```python
from build123d import *

# Parameters (mm, degrees)
F1_W     = 170
F1_H     = 100
F1_R     = 1.75
F2_DEPTH = 5
F3_W     = 5
F3_H     = 5
F3_R     = 1.75
F4_DEPTH = 5


with BuildPart() as f2:
    # F1 (on Top) → F2 (new body)
    with BuildSketch(Plane.XY):
        with Locations((41.5, 26.75)):
            Rectangle(F1_W, F1_H)
        with Locations((14.2, 2.6)):
            Circle(F1_R, mode=Mode.SUBTRACT)
        with Locations((66.5, 7.5)):
            Circle(F1_R, mode=Mode.SUBTRACT)
        with Locations((96.5, 2.6)):
            Circle(F1_R, mode=Mode.SUBTRACT)
        with Locations((15.6, 50.9)):
            Circle(F1_R, mode=Mode.SUBTRACT)
        with Locations((66.5, 35.7)):
            Circle(F1_R, mode=Mode.SUBTRACT)
        with Locations((90.5, 50.9)):
            Circle(F1_R, mode=Mode.SUBTRACT)
    extrude(amount=F2_DEPTH)

    # F3 (on face) → F4 (cut, through all)
    with BuildSketch(Plane.XY.offset(5)):
        with Locations((-26, -20.75)):
            Rectangle(F3_W, F3_H)
        with Locations((-1, -20.75)):
            Rectangle(F3_W, F3_H)
        with Locations((-13.5, -20.75)):
            Circle(F3_R)
        with Locations((84, -20.75)):
            Rectangle(F3_W, F3_H)
        with Locations((96.5, -20.75)):
            Circle(F3_R)
        with Locations((109, -20.75)):
            Rectangle(F3_W, F3_H)
        with Locations((109, 74.25)):
            Rectangle(F3_W, F3_H)
        with Locations((84, 74.25)):
            Rectangle(F3_W, F3_H)
        with Locations((-26, 74.25)):
            Rectangle(F3_W, F3_H)
        with Locations((-13.5, 74.25)):
            Circle(F3_R)
        with Locations((-1, 74.25)):
            Rectangle(F3_W, F3_H)
        with Locations((96.5, 74.25)):
            Circle(F3_R)
        with Locations((-41, 39.25)):
            Rectangle(F3_W, F3_H)
        with Locations((-41, 14.25)):
            Rectangle(F3_W, F3_H)
        with Locations((-41, 26.75)):
            Circle(F3_R)
        with Locations((124, 39.25)):
            Rectangle(F3_W, F3_H)
        with Locations((124, 14.25)):
            Rectangle(F3_W, F3_H)
        with Locations((124, 26.75)):
            Circle(F3_R)
    extrude(amount=-F4_DEPTH, mode=Mode.SUBTRACT)


solid = f2.part
```
Input: part model. Units: mm. Frame: model coordinates. A direction names the side the tool comes from. Coordinates: 2 decimals unless noted, no trailing zeros. Write each loop counter-clockwise with the first axis right and the second up, starting at its lowest first coordinate (ties: lowest second). Pieces come first, ordered by that corner, then holes. Notation, with made-up numbers: (-25, -36.75) -> (-1, -36.75) arc R29 ccw to (-1, -2.75) -> close; hole circle Ø4 at (-11.75, 17.5). An arc over 180 degrees is marked (long way). Answer as a JSON object with one key per item and string values.
1. Mould query, pull axis X, two halves, no side actions, for faces 6 (the face through (-26, 71.75, 3)), 7 (the face through (96, 76.75, 2)), 8 (the face through (-38.5, 39, 3)). Classes: released by +X, released by -X, zero draft, split by the parting line, or undercut.
Result set:
{"face 6": "undercut", "face 7": "zero draft", "face 8": "released by -X"}
2. Section C-C on x = -13.5. Return the cut outline in (y, z).
Result set:
{"outline": "(-23.25, 0) -> (-22.5, 0) -> (-22.5, 5) -> (-23.25, 5) -> close; (-19, 0) -> (72.5, 0) -> (72.5, 5) -> (-19, 5) -> close; (76, 0) -> (76.75, 0) -> (76.75, 5) -> (76, 5) -> close"}
3. Section D-D on y = 26.75. Return the cut outline in (x, z), then the cut area to 3 significant figures.
Result set:
{"outline": "(-43.5, 0) -> (-42.75, 0) -> (-42.75, 5) -> (-43.5, 5) -> close; (-39.25, 0) -> (122.25, 0) -> (122.25, 5) -> (-39.25, 5) -> close; (125.75, 0) -> (126.5, 0) -> (126.5, 5) -> (125.75, 5) -> close", "area": "815 mm2"}
4. Material intervals for line 1 (X direction, y = 2.5, z = 0.3); line 2 (Y direction, x = 96.5, z = 1.6); line 3 (Y direction, x = 83.5, z = 2.3), sorted ascending. Write a range as from..to.
Result set:
{"line 1": "x = -43.5..12.45, 15.95..94.75, 98.25..126.5", "line 2": "y = -23.25..-22.5, -19..0.85, 4.35..72.5, 76..76.75", "line 3": "y = -18.25..71.75"}
5. Access query for faces 1 (the face through (119, -23.25, 2)), 2 (the face through (-38.5, 14, 3)), 3 (the face through (-26, -18.25, 3)), 4 (the face through (124, 16.75, 3)), 5 (the face through (96.272, -19.015, 2.535)). Directions: +Z, -Z, +X, -X, +Y, -Y. A direction counts if a zero-diameter tool reaches every point of the face in a straight line with its end or side. Return the directions, or none.
Result set:
{"face 1": "+Z, -Z, +X, -X, -Y", "face 2": "+Z, -Z, -X", "face 3": "+Z, -Z, -Y", "face 4": "+Z, -Z, +X", "face 5": "+Z, -Z"}
6. First-contact query: P1, Ø3, axis at x = 96.5, y = -20.75, coming from the -Z side; P2, Ø10, axis at x = 44.5, y = 21, coming from the -Z side. Flat tips, straight axial feed; report the tip coordinate or a pass-through.
Result set:
{"P1": "passes through", "P2": "stops at z = 0"}
7. Section B-B on y = -20.75. Return the cut outline in (x, z), then the cut area to 3 significant figures.
Result set:
{"outline": "(-43.5, 0) -> (-28.5, 0) -> (-28.5, 5) -> (-43.5, 5) -> close; (-23.5, 0) -> (-15.25, 0) -> (-15.25, 5) -> (-23.5, 5) -> close; (-11.75, 0) -> (-3.5, 0) -> (-3.5, 5) -> (-11.75, 5) -> close; (1.5, 0) -> (81.5, 0) -> (81.5, 5) -> (1.5, 5) -> close; (86.5, 0) -> (94.75, 0) -> (94.75, 5) -> (86.5, 5) -> close; (98.25, 0) -> (106.5, 0) -> (106.5, 5) -> (98.25, 5) -> close; (111.5, 0) -> (126.5, 0) -> (126.5, 5) -> (111.5, 5) -> close", "area": "715 mm2"}
8. Section A-A on x = 90.5. Return the cut outline in (y, z), then the cut area to 4 significant figures.
Result set:
{"outline": "(-23.25, 0) -> (49.15, 0) -> (49.15, 5) -> (-23.25, 5) -> close; (52.65, 0) -> (76.75, 0) -> (76.75, 5) -> (52.65, 5) -> close", "area": "482.5 mm2"}
